from build123d import *

# Parameters (mm, degrees)
F1_ANGLE      = 180
F3_DEPTH      = 44.6
F3_DEPTH_BACK = 39.8
F4_DEPTH      = 25
F5_DEPTH      = 25
F6_DEPTH      = 152.4


with BuildPart() as f1:
    # F0 (on Top) → F1 (revolve)
    with BuildSketch(Plane.XY):
        Polygon((-31.75, 0), (-29.6666666667, 0), (-74.1166666667, 152.4), (-76.2, 152.4), align=None)
    revolve(axis=Axis((0, 76.2, 0), (0, -1, 0)), revolution_arc=F1_ANGLE)

    # F2 (on Right) → F3 (join, two sides)
    with BuildSketch(Plane.YZ) as f3_sk:
        Polygon((-9.2604166667, -29.0490451389), (0, -31.75), (9.2604166667, 0), (0, 2.7009548611), align=None)
    extrude(amount=F3_DEPTH)
    extrude(f3_sk.sketch, amount=-F3_DEPTH_BACK)

    # F4 (cut): faces of the model
    f4_faces = [f1.faces().sort_by_distance(p)[0] for p in [
        (33.8924298462, 3.5692640267, -19.5125233371),
        (-30.9009295453, 3.1872250967, -20.8223710971),
    ]]
    extrude(f4_faces, amount=-F4_DEPTH, mode=Mode.SUBTRACT)

    # F5 (cut): a face of the model
    f5_faces = [f1.faces().sort_by_distance(p)[0] for p in [
        (0, 5.5929259121, -12.5742540156),
    ]]
    extrude(f5_faces, amount=-F5_DEPTH, mode=Mode.SUBTRACT)

    # F6 (add): a face of the model
    f6_faces = [f1.faces().sort_by_distance(p)[0] for p in [
        (33.4092881944, -0.2139993496, 1.9672428053),
    ]]
    extrude(f6_faces, amount=F6_DEPTH)


solid = f1.part
Could you check a few things on this model? Use its own coordinates, in mm. Coordinates: 2 decimals unless noted, no trailing zeros. Loops run counter-clockwise (first coordinate to the right, second up) from the corner with the lowest first, then second, coordinate; pieces in that order, holes last. Notation, with made-up numbers: (37.25, 74) -> (86.25, 74) arc R18 ccw to (86.25, 100) -> close; hole circle Ø9 at (24, 1). An arc over 180 degrees is marked (long way). Answer in a Markdown table with one row per item.
(1) Will these pins go through, and if not, where does the flat tip stop? pin 1 Ø3 at (y, z) = (11, -23.5) entering from +X; pin 2 Ø4 at (x, y) = (-23, -124.5) entering from -Z; pin 3 Ø3 at (x, y) = (-6, 82.5) entering from -Z.
Results found:
| item | result |
|---|---|
| pin 1 | stops at x = 27.29 |
| pin 2 | stops at z = 12.2 |
| pin 3 | stops at z = -55.96 |
(2) Imagine slicing it at A-A (y = 38). List the corners of the cut face in (x, z) for me, plus the area to 3 significant figures.
Results found:
| item | result |
|---|---|
| outline | (-42.83, 0) arc R42.83 ccw to (42.83, 0) -> (40.75, 0) arc R40.75 cw to (-40.75, 0) -> close |
| area | 274 mm^2 |
(3) If I drill on probe 1 along X at (y, z) = (58.5, -21); probe 2 along X at (y, z) = (122, -2); probe 3 along Z at (x, y) = (-5, -110.5), over which ranges is the centre line in solid material (lowest first)?
Results found:
| item | result |
|---|---|
| probe 1 | x = -44.06 to -41.74, 41.74 to 44.06 |
| probe 2 | x = -67.3 to -65.22, 65.22 to 67.3 |
| probe 3 | z = 0.87 to 2.98 |
(4) Thinking about a two-plate mould opening in X: for faces 1 (the face through (-1.15, 77.54, -52.27)), 2 (the face through (-1.18, 75.13, -53.65)), 3 (the face through (0, 152.4, -75)), which applies, released by +X, released by -X, zero draft, split by the parting line, or undercut?
Results found:
| item | result |
|---|---|
| face 1 | undercut |
| face 2 | split by the parting line |
| face 3 | zero draft |
